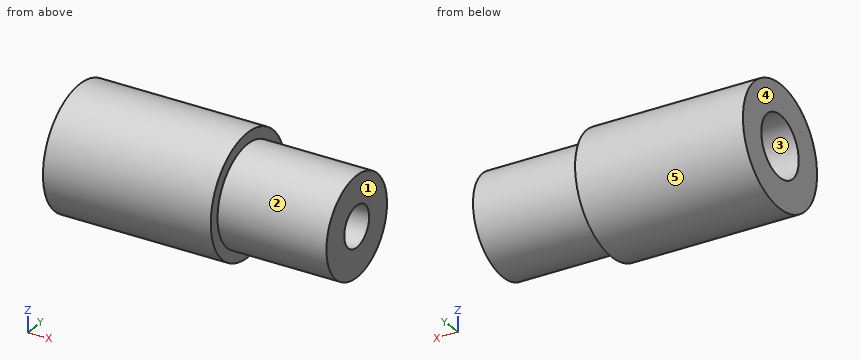
from build123d import *

# Parameters (mm, degrees)
SOCKET_1_SKETCH_W = 17.8
SOCKET_1_SKETCH_H = 4.7625
SOCKET_2_SKETCH_W = 16.2
SOCKET_2_SKETCH_H = 3.175


with BuildPart() as part:
    # Reducer_T6_T4 Sketch → Reducer_T6_T4 (revolve)
    with BuildSketch(Plane.XY, mode=Mode.PRIVATE) as reducer_t6_t4_sk:
        Polygon((-21.6, 0), (-21.6, 9.45), (0.4, 9.45), (4.6, 9.45), (4.6, 7.722), (21.6, 7.722), (21.6, 0), align=None)
    revolve(reducer_t6_t4_sk.sketch.rotate(Axis((-1000, 0, 0), (1, 0, 0)), 90), axis=Axis((-1000, 0, 0), (1, 0, 0)))

    # Socket 1 Sketch → Socket 1 (revolve, cut)
    with BuildSketch(Plane.XY, mode=Mode.PRIVATE) as socket_1_sk:
        with Locations((-13.7, 2.38125)):
            Rectangle(SOCKET_1_SKETCH_W, SOCKET_1_SKETCH_H)
    revolve(socket_1_sk.sketch.rotate(Axis((-1000, 0, 0), (1, 0, 0)), 90), axis=Axis((-1000, 0, 0), (1, 0, 0)), mode=Mode.SUBTRACT)

    # Socket 2 Sketch → Socket 2 (revolve, cut)
    with BuildSketch(Plane.XY, mode=Mode.PRIVATE) as socket_2_sk:
        with Locations((14.5, 1.5875)):
            Rectangle(SOCKET_2_SKETCH_W, SOCKET_2_SKETCH_H)
    revolve(socket_2_sk.sketch.rotate(Axis((-1000, 0, 0), (1, 0, 0)), 90), axis=Axis((-1000, 0, 0), (1, 0, 0)), mode=Mode.SUBTRACT)


solid = part.part
Verification items for the finished model (mm, model axes). Face numbers are marked on the shaded views. A direction names the side the tool comes from. Give positions to 0.01 mm unless a question says otherwise; leave off trailing zeros. Order: outer loops, then holes, each group sorted by start corner. A loop starts at its lowest first (then second) coordinate and runs counter-clockwise, first axis right, second up. Notation, with made-up numbers: M -39.5,64.5 L 0.5,64.5 A27 ccw 0.5,91.5 Z; hole C -23.75,36 d4. An arc over 180 degrees is marked long. Answer as a JSON object with one key per item and string values. Group by question number.
1) Cross-section at D-D (y = -7.25). Enter the section's corners in (x, z).
2) Access from +Z, -Z, +X, -X, +Y, -Y to the whole of each face (thin tool, end or side, straight path). Record for the marked faces 1 and 2.
3) Mould release check, pull along Z, two halves, no side actions. Record for the marked faces 3, 4 and 5: released by +Z, released by -Z, zero draft, split by the parting line, or undercut.
4) Depth check by flat-ended pin: pin 1 Ø8 at (x, z) = (-3.5, -1.5) entering from -Y; pin 2 Ø3 at (y, z) = (0.5, 0.5) entering from +X; pin 3 Ø8 at (x, z) = (9, 2) entering from +Y; pin 4 Ø7.5 at (y, z) = (0, 0) entering from -X. Enter the tip coordinate at first touch or a pass-through.
5) Scan lines: line 1 along Y through (x, z) = (-12.25, 0); line 2 along X through (y, z) = (-1, 2.75); line 3 along X through (y, z) = (5, -6.5). Record each from-to range of solid material in increasing order. Write a range as [from, to].
Result sheet:
{
 "1": {"outline": "M -21.6,-6.06 L 4.6,-6.06 L 4.6,-2.66 L 21.6,-2.66 L 21.6,2.66 L 4.6,2.66 L 4.6,6.06 L -21.6,6.06 Z"},
 "2": {"face 1": "+Z, -Z, +X, +Y, -Y", "face 2": "+X"},
 "3": {"face 3": "undercut", "face 4": "zero draft", "face 5": "split by the parting line"},
 "4": {"pin 1": "stops at y = -9.45", "pin 2": "stops at x = 6.4", "pin 3": "stops at y = 7.72", "pin 4": "stops at x = -4.8"},
 "5": {"line 1": "y = [-9.45, -4.76], [4.76, 9.45]", "line 2": "x = [-4.8, 6.4]", "line 3": "x = [-21.6, 4.6]"}
}
